```python
from build123d import *

# Parameters (mm, degrees)
SKETCH_1_R          = 1.7
EXTRUDE_1_DEPTH     = 3
SKETCH_2_R          = 1.5
SKETCH_2_R_2        = 2
CUT_EXTRUDE_1_DEPTH = 71.242437315
FILLET_1_R          = 5
FILLET_2_R          = 3


with BuildPart() as part:
    # 草图1 → 凸台-拉伸1 (new body)
    with BuildSketch(Plane(origin=(0, 0, 0), x_dir=(1, 0, 0), z_dir=(0, 1, 0))):
        Polygon((0, 0), (0, 30), (39, 30), (39, 38), (59, 38), (59, -38), (39, -38), (39, -30), (0, -30), align=None)
        with Locations(Location((42.5, 25, 0), (0, 0, 270))):
            Circle(SKETCH_1_R, mode=Mode.SUBTRACT)
        with Locations(Location((42.5, -25, 0), (0, 0, 270))):
            Circle(SKETCH_1_R, mode=Mode.SUBTRACT)
        with Locations(Location((42.5, 0, 0), (0, 0, 270))):
            Circle(SKETCH_1_R, mode=Mode.SUBTRACT)
        with Locations(Location((53, 30, 0), (0, 0, 270))):
            Circle(SKETCH_1_R, mode=Mode.SUBTRACT)
        with Locations(Location((53, 0, 0), (0, 0, 270))):
            Circle(SKETCH_1_R, mode=Mode.SUBTRACT)
        with Locations(Location((53, -30, 0), (0, 0, 270))):
            Circle(SKETCH_1_R, mode=Mode.SUBTRACT)
    extrude(amount=EXTRUDE_1_DEPTH)

    # 草图2 → 切除-拉伸1 (cut, through all)
    with BuildSketch(Plane(origin=(0, 3, 0), x_dir=(1, 0, 0), z_dir=(0, 1, 0))):
        with Locations(Location((32.5, 0.5, 0), (0, 0, 270))):
            Circle(SKETCH_2_R)
        with Locations(Location((5, 0.5, 0), (0, 0, 270))):
            Circle(SKETCH_2_R_2)
        with Locations(Location((5, 10.5, 0), (0, 0, 270))):
            Circle(SKETCH_2_R_2)
        with Locations(Location((53, 10.5, 0), (0, 0, 270))):
            Circle(SKETCH_2_R_2)
        with Locations(Location((29, 18, 0), (0, 0, 270))):
            Circle(SKETCH_2_R)
        with Locations(Location((18.5, -6.5, 0), (0, 0, 270))):
            Circle(SKETCH_2_R)
        with Locations(Location((11.5, 0.5, 0), (0, 0, 270))):
            Circle(SKETCH_2_R)
        with Locations(Location((25.5, 0.5, 0), (0, 0, 270))):
            Circle(SKETCH_2_R)
        with Locations(Location((18.5, 7.5, 0), (0, 0, 270))):
            Circle(SKETCH_2_R)
    extrude(amount=-CUT_EXTRUDE_1_DEPTH, mode=Mode.SUBTRACT)

    # 圆角1
    fillet_1_edges = [part.edges().sort_by_distance(p)[0] for p in [
        (59, 1.5, 38),
        (39, 1.5, 30),
        (0, 1.5, 30),
        (0, 1.5, -30),
        (39, 1.5, -30),
        (59, 1.5, -38),
    ]]
    fillet(fillet_1_edges, radius=FILLET_1_R)

    # 圆角2
    fillet_2_edges = [part.edges().sort_by_distance(p)[0] for p in [
        (39, 1.5, 38),
        (39, 1.5, -38),
    ]]
    fillet(fillet_2_edges, radius=FILLET_2_R - 0.0001)  # a hair under: the kernel refuses the full size


solid = part.part
```
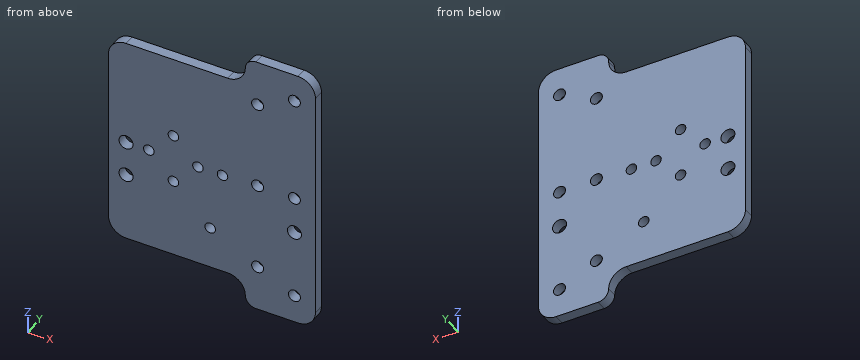
Could you check a few things on this model? Use its own coordinates, in mm. Coordinates: 2 decimals unless noted, no trailing zeros. Order: outer loops, then holes, each group sorted by start corner. A loop starts at its lowest first (then second) coordinate and runs counter-clockwise, first axis right, second up. Notation, with made-up numbers: M 8,-5 L 27,-5 A19 ccw 27,10 Z; hole C 65.5,39 d5. An arc over 180 degrees is marked long. Use one line per item in the form item = value. Start each with the question number.
1. Suppose I cut it at C-C on z = 6.5. Write out the boundary of the cut face in (x, y), then the cut area to 3 significant figures.
2. Suppose I cut it at D-D on x = 53. Write out the boundary of the cut face in (y, z).
3. Suppose I cut it at B-B on x = 29. Write out the boundary of the cut face in (y, z), then the cut area to 3 significant figures.
4. For pin 1 (4.5 mm diameter, centred on x = 53, z = -10.5, fed in from +Y), with a flat end and sliding along its axis, tell me the tip position at first contact or that it passes through.
5. Suppose I cut it at A-A on z = -10.5. Write out the boundary of the cut face in (x, y), then the cut area to 3 significant figures.
6. Please list where these lines run through material, in increasing order: line 1 (X direction, y = 1.1, z = -25); line 2 (X direction, y = 1.1, z = -7.5); line 3 (Z direction, x = 4, y = 0.6).
Geometry says:
q1.outline = M 0,0 L 17,0 L 17,3 L 0,3 Z; M 20,0 L 59,0 L 59,3 L 20,3 Z
q1.area = 168 mm^2
q2.outline = M 0,-38 L 3,-38 L 3,-31.7 L 0,-31.7 Z; M 0,-28.3 L 3,-28.3 L 3,-12.5 L 0,-12.5 Z; M 0,-8.5 L 3,-8.5 L 3,-1.7 L 0,-1.7 Z; M 0,1.7 L 3,1.7 L 3,28.3 L 0,28.3 Z; M 0,31.7 L 3,31.7 L 3,38 L 0,38 Z
q3.outline = M 0,-30 L 3,-30 L 3,-19.5 L 0,-19.5 Z; M 0,-16.5 L 3,-16.5 L 3,30 L 0,30 Z
q3.area = 171 mm^2
q4.pin_1 = 3
q5.outline = M 0,0 L 3,0 L 3,3 L 0,3 Z; M 7,0 L 51,0 L 51,3 L 7,3 Z; M 55,0 L 59,0 L 59,3 L 55,3 Z
q5.area = 153 mm^2
q6.line_1 = 0 to 40.8, 44.2 to 59
q6.line_2 = 0 to 17, 20 to 59
q6.line_3 = -29.9 to -12.23, -8.77 to -2.23, 1.23 to 29.9
